Read the model definition and answer for the solid it produces. Units are mm, in the model's axes. A direction names the side the tool comes from. Coordinates: 2 decimals unless noted, no trailing zeros. Write each loop counter-clockwise with the first axis right and the second up, starting at its lowest first coordinate (ties: lowest second). Pieces come first, ordered by that corner, then holes. Notation, with made-up numbers: (14.25, 87) - (68.25, 87) arc R28 cw to (68.25, 124) - close; hole circle Ø10 at (14.25, 2). An arc over 180 degrees is marked (long way). Return JSON: item names as keys, results as strings.
Autodesk Inventor part; units mm, degrees
ref_plane "Work Plane1" through (0, 15, 0) normal (0, 1, 0) x (-1, 0, 0)
ref_plane "YZ Plane" through (0, 0, 0) normal (1, 0, 0) x (0, 1, 0)
ref_plane "XY Plane" through (0, 0, 0) normal (0, 0, 1) x (1, 0, 0)
sketch "Sketch1" plane through (0, 0, 0) normal (0, 0, 1) x (1, 0, 0)
  circle A0 centre (0, 0) radius 19.05
  dimension "d0" = 38.1
extrude "Extrusion1" add sketch "Sketch1" along normal blind 480
ref_plane "Work Plane1" through (0, 15, 0) normal (0, 1, 0) x (-1, 0, 0)
sketch "Sketch2" plane through (0, 15, 0) normal (0, 1, 0) x (-1, 0, 0)
  line L0 (-122.6999, 230) -> (112.1399, 230) construction
  line L1 (-19.05, 0) -> (19.05, 0)
  line L2 (-122.6999, 128) -> (109.8048, 128) construction
  line L3 (-29.6313, 106) -> (33.0816, 106)
  line L4 (33.0816, 106) -> (33.0816, 118)
  line L5 (33.0816, 118) -> (-29.6313, 118)
  line L6 (-29.6313, 118) -> (-29.6313, 106)
  line L7 (-41.3065, 342) -> (43.7561, 342)
  line L8 (43.7561, 342) -> (43.7561, 354)
  line L9 (43.7561, 354) -> (-41.3065, 354)
  line L10 (-41.3065, 354) -> (-41.3065, 342)
  point P0 (0, 0)
  dimension "d5" = 230
  dimension "d6" = 102
  dimension "d8" = 12
  dimension "d9" = 12
  dimension "d11" = 112
  dimension "d14" = 112
extrude "Extrusion2" cut sketch "Sketch2" along normal through all
properties part number "1231_Spool Shaft_V1" material "Iron, Ductile"
(1) Flat-ended cylindrical pins translate along their axes: P1, Ø5, axis at y = -14.5, z = 385.5, coming from the +X side; P2, Ø6, axis at x = 1, z = 348, coming from the +Y side; P3, Ø4, axis at y = 13, z = 65.5, coming from the -X side; P4, Ø3, axis at x = 1.5, y = 17, coming from the -Z side. Find the tip coordinate at first contact, or state that the pin passes through.
Answer:
{"P1": "x = 14.8", "P2": "y = 15", "P3": "x = -15.55", "P4": "z = 0"}
(2) A cutting plane is placed at C-C (y = -12.5). Determine the outline of the cut face in (x, z), and give its area (3 significant figures).
Answer:
{"outline": "(-14.38, 0) - (14.38, 0) - (14.38, 480) - (-14.38, 480) - close", "area": "13,800 mm²"}
(3) Straight lines are drawn through the part: line 1 (Y direction, x = 0, z = 96); line 2 (Y direction, x = 9, z = 461.5); line 3 (X direction, y = 7, z = 211). For each, find the intervals that lie inside material, in ascending order. Write a range as from..to.
Answer:
{"line 1": "-19.05..19.05", "line 2": "-16.79..16.79", "line 3": "-17.72..17.72"}
(4) Which of the six approach directions +Z, -Z, +X, -X, +Y, -Y give full straight-line access (tool end or side, diameter ignored) to faces 1 (the face through (-2.48, -18.888, 236.64)), 2 (the face through (0, 15, 348))?
Answer:
{"face 1": "+Z, -Z", "face 2": "+X, -X, +Y"}
(5) A cutting plane is placed at B-B (z = 268.5). Determine the outline of the cut face in (x, y).
Answer:
{"outline": "circle Ø38.1 at (0, 0)"}
(6) A cutting plane is placed at A-A (x = -3.5). Determine the outline of the cut face in (y, z).
Answer:
{"outline": "(-18.73, 0) - (18.73, 0) - (18.73, 106) - (15, 106) - (15, 118) - (18.73, 118) - (18.73, 342) - (15, 342) - (15, 354) - (18.73, 354) - (18.73, 480) - (-18.73, 480) - close"}
